Model file for the job. Use its own axes, mm. A direction names the side the tool comes from. Give positions to 0.01 mm unless a question says otherwise; leave off trailing zeros. Write each loop counter-clockwise with the first axis right and the second up, starting at its lowest first coordinate (ties: lowest second). Pieces come first, ordered by that corner, then holes. Notation, with made-up numbers: (2, 75.5) - (38, 75.5) arc R21 cw to (38, 101.5) - close; hole circle Ø4 at (-30.5, 43.5). An arc over 180 degrees is marked (long way). Use CSV: the item, a comma, the result in double quotes.
from build123d import *

# Parameters (mm, degrees)
F1_DEPTH = 30
F4_R     = 2.5
F5_DEPTH = 50
F6_R     = 2.75
F7_DEPTH = 25


with BuildPart() as f1:
    # F0 (on Front) → F1 (new body)
    with BuildSketch(Plane.XZ):
        with BuildLine():
            Line((9.5, 0), (12, 0))
            ThreePointArc((12, 0), (0, 12), (-12, 0))
            Line((-12, 0), (-9.5, 0))
            ThreePointArc((-9.5, 0), (0, 9.5), (9.5, 0))
        make_face()
        with BuildLine():
            Line((12, -24), (12, 0))
            ThreePointArc((12, 0), (11.3578166916, -3.8729833462), (9.5, -7.3314391493))
            Line((9.5, -7.3314391493), (9.5, -24))
            Line((9.5, -24), (12, -24))
        make_face()
        with BuildLine():
            ThreePointArc((9.5, -7.3314391493), (11.3578166916, -3.8729833462), (12, 0))
            Line((12, 0), (9.5, 0))
            Line((9.5, 0), (9.5, -7.3314391493))
        make_face()
        with BuildLine():
            Line((-9.5, 0), (-12, 0))
            ThreePointArc((-12, 0), (-11.3578166916, -3.8729833462), (-9.5, -7.3314391493))
            Line((-9.5, -7.3314391493), (-9.5, 0))
        make_face()
        with BuildLine():
            ThreePointArc((-9.5, -7.3314391493), (-11.3578166916, -3.8729833462), (-12, 0))
            Line((-12, 0), (-12, -24))
            Line((-12, -24), (-9.5, -24))
            Line((-9.5, -24), (-9.5, -7.3314391493))
        make_face()
        with BuildLine():
            ThreePointArc((-9.5, -7.3314391493), (0, -12), (9.5, -7.3314391493))
            Line((9.5, -7.3314391493), (9.5, 0))
            ThreePointArc((9.5, 0), (0, -9.5), (-9.5, 0))
            Line((-9.5, 0), (-9.5, -7.3314391493))
        make_face()
    extrude(amount=F1_DEPTH)

    # F3: sweep along a path in F2
    with BuildLine(Plane.YZ) as f3_path:
        ThreePointArc((0, 0), (17.3034739964, 3.4597810832), (31.9462265702, 13.3071205486))
    # F0 (on Front) → F3 (sweep)
    with BuildSketch(Plane.XZ):
        with BuildLine():
            Line((9.5, 0), (12, 0))
            ThreePointArc((12, 0), (0, 12), (-12, 0))
            Line((-12, 0), (-9.5, 0))
            ThreePointArc((-9.5, 0), (0, 9.5), (9.5, 0))
        make_face()
        with BuildLine():
            ThreePointArc((9.5, -7.3314391493), (11.3578166916, -3.8729833462), (12, 0))
            Line((12, 0), (9.5, 0))
            Line((9.5, 0), (9.5, -7.3314391493))
        make_face()
        with BuildLine():
            ThreePointArc((-9.5, -7.3314391493), (0, -12), (9.5, -7.3314391493))
            Line((9.5, -7.3314391493), (9.5, 0))
            ThreePointArc((9.5, 0), (0, -9.5), (-9.5, 0))
            Line((-9.5, 0), (-9.5, -7.3314391493))
        make_face()
        with BuildLine():
            Line((-9.5, 0), (-12, 0))
            ThreePointArc((-12, 0), (-11.3578166916, -3.8729833462), (-9.5, -7.3314391493))
            Line((-9.5, -7.3314391493), (-9.5, 0))
        make_face()
    sweep(path=f3_path.line)

    # F4 (on face) → F5 (cut)
    with BuildSketch(Plane.YZ.offset(12)):
        with Locations((-25, -17.2888711095)):
            Circle(F4_R)
        with Locations((-5, -17.2888711095)):
            Circle(F4_R)
    extrude(amount=-F5_DEPTH, mode=Mode.SUBTRACT)

    # F6 (on Top) → F7 (cut)
    with BuildSketch(Plane.XY):
        with Locations((0, -21.25)):
            Circle(F6_R)
    extrude(amount=F7_DEPTH, mode=Mode.SUBTRACT)


solid = f1.part
(1) Wall check: probe 1 along Y at (x, z) = (9.75, -17); probe 2 along Z at (x, y) = (0, -13.5); probe 3 along Z at (x, y) = (-7.25, -9.5). Give the ranges that are in metal, low to high. Write a range as [from, to].
Checked values:
probe 1,"y = [-30, -27.48], [-22.52, -7.48], [-2.52, 0]"
probe 2,"z = [-12, -9.5], [9.5, 12]"
probe 3,"z = [-9.56, -6.14], [6.14, 9.56]"
(2) Saw through at C-C, the plane y = -16. List the corners of the cut face in (x, z), then the cut area to 3 significant figures.
Checked values:
outline,"(-12, -24) - (-9.5, -24) - (-9.5, -7.33) arc R12 ccw to (9.5, -7.33) - (9.5, -24) - (12, -24) - (12, 0) arc R12 ccw to (-12, 0) - close; hole circle Ø19 at (0, 0)"
area,"264 mm^2"
(3) Flat gauge pins, fed straight in: P1, Ø1, axis at x = 0, z = 2.5, coming from the -Y side; P2, Ø1.5, axis at x = -5.5, y = 30, coming from the -Z side; P3, Ø7, axis at x = 0, y = -21.25, coming from the +Z side. Where does each tip first touch, or does it go through?
Checked values:
P1,"stops at y = 33.49"
P2,"stops at z = -2.53"
P3,"stops at z = 12"
(4) Pull direction Y, two halves, no side cores. Call faces 1 (the face through (10.768, -26.984, -18.81)), 2 (the face through (-12, -15, -12)), 3 (the face through (-1, -30, -10)), 4 (the face through (-9.834, 31.355, 13.894)): released by +Y, released by -Y, zero draft, split by the parting line, or undercut.
Checked values:
face 1,"undercut"
face 2,"zero draft"
face 3,"released by -Y"
face 4,"released by +Y"
(5) Saw through at A-A, the plane y = -5. List the corners of the cut face in (x, z), then the cut area to 3 significant figures.
Checked values:
outline,"(-12, -24) - (-9.5, -24) - (-9.5, -19.79) - (-12, -19.79) - close; (-12, -14.79) - (-9.5, -14.79) - (-9.5, -7.33) arc R12 ccw to (9.5, -7.33) - (9.5, -14.79) - (12, -14.79) - (12, 0) arc R12 ccw to (-12, 0) - close; (9.5, -24) - (12, -24) - (12, -19.79) - (9.5, -19.79) - close; hole circle Ø19 at (0, 0)"
area,"239 mm^2"
(6) Saw through at D-D, the plane x = -1.75. List the corners of the cut face in (y, z).
Checked values:
outline,"(-30, -11.87) - (0, -11.87) arc R56.87 ccw to (40.37, 4.95) - (38.58, 6.73) arc R54.34 cw to (0, -9.34) - (-30, -9.34) - close; (-30, 9.34) - (-23.37, 9.34) - (-23.37, 11.87) - (-30, 11.87) - close; (-19.13, 9.34) - (0, 9.34) arc R35.66 ccw to (25.32, 19.88) - (23.52, 21.67) arc R33.13 cw to (0, 11.87) - (-19.13, 11.87) - close"
(7) 3-axis set-ups, long thin cutter, end or side, ignore diameter. For faces 5 (the face through (1.48, -18.93, 10.53)), 6 (the face through (11, 0, -14)), 7 (the face through (9.5, -15, -16)), 8 (the face through (-11, 0, -14)): which of +Z, -Z, +X, -X, +Y, -Y reach the whole face in a straight line?
Checked values:
face 5,"+Z"
face 6,"-Z, +X, +Y"
face 7,"-Z, +Y, -Y"
face 8,"-Z, -X, +Y"
(8) Saw through at B-B, the plane z = -20.5. List the corners of the cut face in (x, y).
Checked values:
outline,"(-12, -30) - (-9.5, -30) - (-9.5, 0) - (-12, 0) - close; (9.5, -30) - (12, -30) - (12, 0) - (9.5, 0) - close"
